Geometry check sheet. Reference: drawing and pictorial views, mm from the part's lowest x, y, z. Round coordinates to 2 decimals unless told otherwise and drop trailing zeros. Order: outer loops, then holes, each group sorted by start corner. A loop starts at its lowest first (then second) coordinate and runs counter-clockwise, first axis right, second up.
(1) Go/stop test with flat-tipped pins: pin 1 (0.6 mm diameter, centred on x = 0.5, z = 21.5, fed in from +Y); pin 2 (2 mm diameter, centred on x = 0.5, z = 15.5, fed in from -Y). Record where each tip stops, or that it passes through.
(2) Material ranges on line 1 along Y through (x, z) = (0.45, 28.5); line 2 along Y through (x, z) = (2.25, 39), recorded low to high.
(3) Sectioned sample at A-A (z = 11). Record the boundary of the cut face in (x, y), plus the area to 3 significant figures.
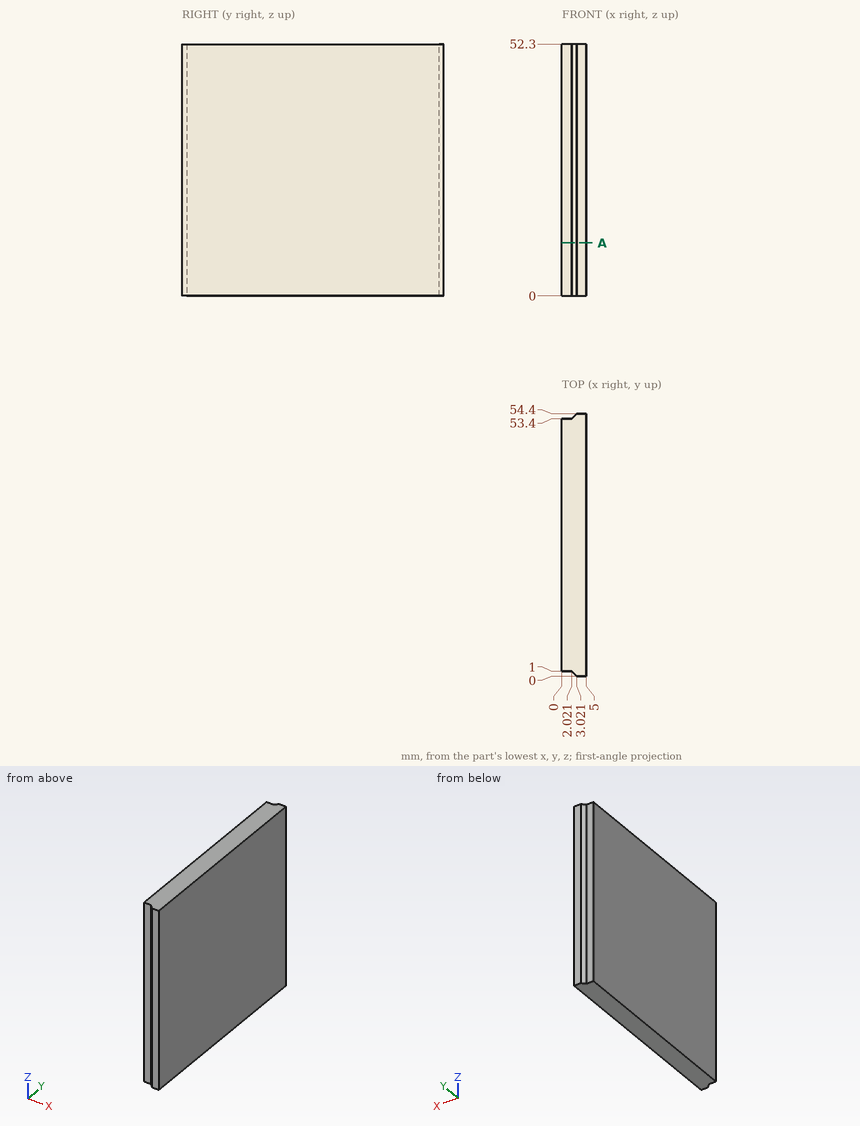
Answer below:
1. pin 1: stops at y = 53.4
1. pin 2: stops at y = 1
2. line 1: y = 1 to 53.4
2. line 2: y = 0.77 to 53.63
3. outline: (0, 1) - (2.02, 1) - (3.02, 0) - (5, 0) - (5, 54.4) - (3.02, 54.4) - (2.02, 53.4) - (0, 53.4) - close
3. area: 267 mm2
